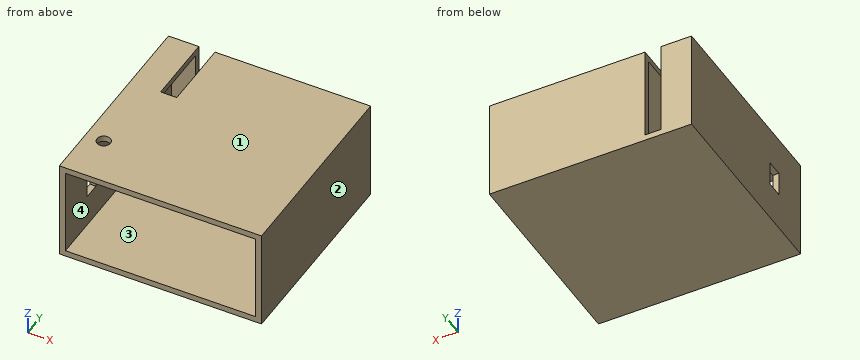
from build123d import *

# Parameters (mm, degrees)
SKETCH1_W           = 100
SKETCH1_H           = 100
BOSS_EXTRUDE2_DEPTH = 50
SKETCH3_W           = 8
SKETCH3_H           = 35
CUT_EXTRUDE2_DEPTH  = 47
SKETCH4_W           = 94
SKETCH4_H           = 44
CUT_EXTRUDE3_DEPTH  = 97
CUT_EXTRUDE4_REACH  = 152
SKETCH5_W           = 12
SKETCH5_H           = 8
CUT_EXTRUDE5_REACH  = 152
SKETCH6_R           = 3.35


with BuildPart() as part:
    # Sketch1 → Boss-Extrude2 (new body)
    with BuildSketch(Plane.XY):
        with Locations((50, 50)):
            Rectangle(SKETCH1_W, SKETCH1_H)
    extrude(amount=-BOSS_EXTRUDE2_DEPTH)

    # Sketch3 → Cut-Extrude2 (cut)
    with BuildSketch(Plane.XY):
        with Locations((19, 82.5)):
            Rectangle(SKETCH3_W, SKETCH3_H)
    extrude(amount=-CUT_EXTRUDE2_DEPTH, mode=Mode.SUBTRACT)

    # Sketch4 → Cut-Extrude3 (cut)
    with BuildSketch(Plane.XZ):
        with Locations((50, -25)):
            Rectangle(SKETCH4_W, SKETCH4_H)
    extrude(amount=-CUT_EXTRUDE3_DEPTH, mode=Mode.SUBTRACT)

    # Sketch5 → Cut-Extrude4 (cut, up to next)
    with BuildSketch(Plane.ZY, mode=Mode.PRIVATE) as cut_extrude4_sk1:
        with Locations((-25, 24)):
            Rectangle(SKETCH5_W, SKETCH5_H)
    cut_extrude4_tool1 = extrude(cut_extrude4_sk1.sketch, amount=-CUT_EXTRUDE4_REACH, mode=Mode.PRIVATE) & part.part
    add(cut_extrude4_tool1.solids().sort_by_distance((0, 24, -25))[0], mode=Mode.SUBTRACT)

    # Sketch6 → Cut-Extrude5 (cut, up to next)
    with BuildSketch(Plane.XY, mode=Mode.PRIVATE) as cut_extrude5_sk1:
        with Locations((9, 24)):
            Circle(SKETCH6_R)
    cut_extrude5_tool1 = extrude(cut_extrude5_sk1.sketch, amount=-CUT_EXTRUDE5_REACH, mode=Mode.PRIVATE) & part.part
    add(cut_extrude5_tool1.solids().sort_by_distance((9, 24, 0))[0], mode=Mode.SUBTRACT)


solid = part.part
The listing builds one solid part. Answer for the finished solid, in the listing's coordinates (mm). Face numbers are marked on the shaded views. Give positions to 0.01 mm unless a question says otherwise; leave off trailing zeros. Order: outer loops, then holes, each group sorted by start corner. A loop starts at its lowest first (then second) coordinate and runs counter-clockwise, first axis right, second up. Notation, with made-up numbers: (86.25, 14) - (127.25, 14) arc R24 ccw to (127.25, 26) - close; hole circle Ø3 at (8.5, 63.25). An arc over 180 degrees is marked (long way). Use one line per item in the form item = value.
1) Find section C-C on y = 43.5. Determine the outline of the cut face in (x, z), and give its area (3 significant figures).
Verdict:
outline = (0, -50) - (100, -50) - (100, 0) - (0, 0) - close; hole (3, -47) - (97, -47) - (97, -3) - (3, -3) - close
area = 864 mm^2
2) Find section B-B on y = 24. Determine the outline of the cut face in (x, z).
Verdict:
outline = (0, -50) - (100, -50) - (100, 0) - (12.35, 0) - (12.35, -3) - (97, -3) - (97, -47) - (3, -47) - (3, -31) - (0, -31) - close; (0, -19) - (3, -19) - (3, -3) - (5.65, -3) - (5.65, 0) - (0, 0) - close
3) The mould has two halves that part along X. Classify the marked faces 1, 2, 3 and 4: released by +X, released by -X, zero draft, split by the parting line, or undercut.
Verdict:
face_1 = zero draft
face_2 = released by +X
face_3 = undercut
face_4 = undercut
4) Consider probe 1 along Z at (x, y) = (37.5, 62.5); probe 2 along Y at (x, z) = (9, -2.2); probe 3 along X at (y, z) = (7, -31). Determine where each line is inside the solid, lowest interval first. Write a range as [from, to].
Verdict:
probe_1 = [-50, -47], [-3, 0]
probe_2 = [0, 20.65], [27.35, 100]
probe_3 = [0, 3], [97, 100]
5) Each of these flat-tipped pins is pushed along its axis until it touches: pin 1 (1.5 mm diameter, centred on x = 18, z = -1, fed in from +Y); pin 2 (22 mm diameter, centred on x = 41.5, z = -21, fed in from -Y). Where does it stop, or does it pass through?
Verdict:
pin_1 = 65
pin_2 = 97
6) Find section A-A on x = 9. Determine the outline of the cut face in (y, z).
Verdict:
outline = (0, -50) - (100, -50) - (100, 0) - (27.35, 0) - (27.35, -3) - (97, -3) - (97, -47) - (0, -47) - close; (0, -3) - (20.65, -3) - (20.65, 0) - (0, 0) - close
7) Find section D-D on z = -7. Determine the outline of the cut face in (x, y).
Verdict:
outline = (0, 0) - (3, 0) - (3, 97) - (15, 97) - (15, 100) - (0, 100) - close; (23, 97) - (97, 97) - (97, 0) - (100, 0) - (100, 100) - (23, 100) - close
